Could you check a few things on this model? Use its own coordinates, in mm. A direction names the side the tool comes from. Coordinates: 2 decimals unless noted, no trailing zeros. Loops run counter-clockwise (first coordinate to the right, second up) from the corner with the lowest first, then second, coordinate; pieces in that order, holes last.
from build123d import *

# Parameters (mm, degrees)
SKETCH_1_R          = 3
SKETCH_1_R_2        = 1.5
EXTRUDE_1_DEPTH     = 25
EXTRUDE_2_DEPTH     = 5
SKETCH_3_R          = 1.5
CUT_EXTRUDE_1_DEPTH = 26
SKETCH_4_R          = 5
CUT_EXTRUDE_2_DEPTH = 4
SKETCH_5_R          = 1.5
EXTRUDE_3_DEPTH     = 5
SKETCH_6_R          = 5
CUT_EXTRUDE_3_DEPTH = 4
SKETCH_7_W          = 8
SKETCH_7_H          = 3
CUT_EXTRUDE_4_DEPTH = 25
SKETCH_8_R          = 1.5
CUT_EXTRUDE_5_DEPTH = 26
SKETCH_9_W          = 62.045271576
SKETCH_9_H          = 47.186533399
CUT_EXTRUDE_6_DEPTH = 2
SKETCH_10_R         = 43.321303534
CUT_EXTRUDE_7_DEPTH = 2


with BuildPart() as part:
    # 草图1 → 凸台-拉伸1 (new body)
    with BuildSketch(Plane.XY):
        with BuildLine():
            Line((-60, -3), (0, -3))
            ThreePointArc((0, -3), (-2.93041003, -0.642415018), (-1.255026274, 2.72486863))
            Line((-1.255026274, 2.72486863), (-5, 1))
            Line((-5, 1), (-60, 1))
            Line((-60, 1), (-60, -3))
        make_face()
        Circle(SKETCH_1_R)
        Circle(SKETCH_1_R_2, mode=Mode.SUBTRACT)
    extrude(amount=EXTRUDE_1_DEPTH)

    # 草图2 → 凸台-拉伸2 (add)
    with BuildSketch(Plane.XY.offset(25)):
        with BuildLine():
            Line((-60, -3), (-60, -19))
            Line((-60, -19), (-48, -19))
            Line((-48, -19), (-48, -14))
            ThreePointArc((-48, -14), (-46.535533906, -10.464466094), (-43, -9))
            Line((-43, -9), (-38, -9))
            ThreePointArc((-38, -9), (-34.464466094, -10.464466094), (-33, -14))
            Line((-33, -14), (-33, -23))
            Line((-33, -23), (-15, -23))
            Line((-15, -23), (-15, -13))
            Line((-15, -13), (-5, -3))
            Line((-5, -3), (-60, -3))
        make_face()
    extrude(amount=-EXTRUDE_2_DEPTH)

    # 草图3 → 切除-拉伸1 (cut, through all)
    with BuildSketch(Plane.XY.offset(25)):
        with Locations((-55, -14)):
            Circle(SKETCH_3_R)
        with Locations((-23, -14)):
            Circle(SKETCH_3_R)
    extrude(amount=-CUT_EXTRUDE_1_DEPTH, mode=Mode.SUBTRACT)

    # 草图4 → 切除-拉伸2 (cut)
    with BuildSketch(Plane.XY.offset(25)):
        Circle(SKETCH_4_R)
    extrude(amount=-CUT_EXTRUDE_2_DEPTH, mode=Mode.SUBTRACT)

    # 草图5 → 凸台-拉伸3 (add)
    with BuildSketch(Plane(origin=(0, 0, 0), x_dir=(-1, 0, 0), z_dir=(0, 0, -1))):
        with BuildLine():
            Line((60, -3), (5, -3))
            Line((5, -3), (15, -13))
            Line((15, -13), (15, -23))
            Line((15, -23), (33, -23))
            Line((33, -23), (33, -14))
            ThreePointArc((33, -14), (34.464466094, -10.464466094), (38, -9))
            Line((38, -9), (43, -9))
            ThreePointArc((43, -9), (46.535533906, -10.464466094), (48, -14))
            Line((48, -14), (48, -19))
            Line((48, -19), (60, -19))
            Line((60, -19), (60, -3))
        make_face()
        with Locations((23, -14)):
            Circle(SKETCH_5_R, mode=Mode.SUBTRACT)
        with Locations((55, -14)):
            Circle(SKETCH_5_R, mode=Mode.SUBTRACT)
    extrude(amount=-EXTRUDE_3_DEPTH)

    # 草图6 → 切除-拉伸3 (cut)
    with BuildSketch(Plane(origin=(0, 0, 0), x_dir=(-1, 0, 0), z_dir=(0, 0, -1))):
        Circle(SKETCH_6_R)
    extrude(amount=-CUT_EXTRUDE_3_DEPTH, mode=Mode.SUBTRACT)

    # 草图7 → 切除-拉伸4 (cut, through all)
    with BuildSketch(Plane(origin=(0, 1, 0), x_dir=(1, 0, 0), z_dir=(0, 1, 0))):
        with Locations((-56, -6.5)):
            Rectangle(SKETCH_7_W, SKETCH_7_H)
        with Locations((-56, -18.5)):
            Rectangle(SKETCH_7_W, SKETCH_7_H)
    extrude(amount=-CUT_EXTRUDE_4_DEPTH, mode=Mode.SUBTRACT)

    # 草图8 → 切除-拉伸5 (cut, through all)
    with BuildSketch(Plane(origin=(0, 0, 0), x_dir=(-1, 0, 0), z_dir=(0, 0, -1))):
        with Locations((58, -1)):
            Circle(SKETCH_8_R)
    extrude(amount=-CUT_EXTRUDE_5_DEPTH, mode=Mode.SUBTRACT)

    # 草图9 → 切除-拉伸6 (cut)
    with BuildSketch(Plane(origin=(0, 0, 0), x_dir=(-1, 0, 0), z_dir=(0, 0, -1))):
        with Locations((33.21865334, -9.347420282)):
            Rectangle(SKETCH_9_W, SKETCH_9_H)
    extrude(amount=-CUT_EXTRUDE_6_DEPTH, mode=Mode.SUBTRACT)

    # 草图10 → 切除-拉伸7 (cut)
    with BuildSketch(Plane.XY.offset(25)):
        with Locations((-29.013307515, -5.864856676)):
            Circle(SKETCH_10_R)
    extrude(amount=-CUT_EXTRUDE_7_DEPTH, mode=Mode.SUBTRACT)


solid = part.part
(1) Imagine slicing it at A-A, the plane x = -58. Write out the boundary of the cut face in (y, z).
Answers:
outline: (-19, 2) - (-2.5, 2) - (-2.5, 5) - (-19, 5) - close; (-19, 20) - (-2.5, 20) - (-2.5, 23) - (-19, 23) - close; (-3, 8) - (-2.5, 8) - (-2.5, 17) - (-3, 17) - close; (0.5, 2) - (1, 2) - (1, 5) - (0.5, 5) - close; (0.5, 8) - (1, 8) - (1, 17) - (0.5, 17) - close; (0.5, 20) - (1, 20) - (1, 23) - (0.5, 23) - close
(2) Which directions (+Z, -Z, +X, -X, +Y, -Y) give clear straight access to the entire face, cutting with the end or side of a thin tool? Please do faces 4 (the face through (-4.878, -1.1, 2.986)), 5 (the face through (-47, -11, 22)), 6 (the face through (-55, -1, 17)), 7 (the face through (-4.9, -1, 22)), 8 (the face through (-32, 1, 12)).
Answers:
face 4: -Z, +X
face 5: +Z, -Z, -Y
face 6: -X, +Y, -Y
face 7: +Z, +X
face 8: +Z, -Z, -X, +Y
(3) For pin 1 (2.5 mm diameter, centred on y = -17.5, z = 21, fed in from +X); pin 2 (3.5 mm diameter, centred on x = -52.5, z = 21, fed in from -Y); pin 3 (3 mm diameter, centred on x = -40.5, z = 19, fed in from +Y), each with a flat end and sliding along its axis, tell me the tip position at first contact or that it passes through.
Answers:
pin 1: stops at x = -15
pin 2: stops at y = -19
pin 3: stops at y = 1
(4) Imagine slicing it at C-C, the plane z = 14.25. Write out the boundary of the cut face in (x, y), and give its area (3 significant figures).
Answers:
outline: (-60, -3) - (0, -3) arc R3 ccw (long way) to (-1.26, 2.72) - (-5, 1) - (-60, 1) - close; hole circle Ø3 at (-58, -1); hole circle Ø3 at (0, 0)
area: 246 mm2
(5) Imagine slicing it at D-D, the plane x = -39.5. Write out the boundary of the cut face in (y, z).
Answers:
outline: (-9, 2) - (1, 2) - (1, 23) - (-9, 23) - (-9, 20) - (-3, 20) - (-3, 5) - (-9, 5) - close
(6) I need wall thicknesses on probe 1 along Z at (x, y) = (-25.5, -16.5); probe 2 along Y at (x, z) = (-55, 3.6); probe 3 along X at (y, z) = (-0.5, 9). Which ranges of each line are inside material? Lowest first, please.
Answers:
probe 1: z = 2 to 5, 20 to 23
probe 2: y = -19 to -15.5, -12.5 to 1
probe 3: x = -60 to -59.41, -56.59 to -1.41, 1.41 to 2.96
(7) We'd pull the mould along Y, two halves only. Please class faces 1 (the face through (-35, -10, 22)), 2 (the face through (-32, -8, 2)), 3 (the face through (-56.43, -13.55, 3.48)): +Y half, -Y half, draft (parallel to the pull), parting line (faces both ways), or undercut.
Answers:
face 1: -Y half
face 2: draft
face 3: undercut
(8) Imagine slicing it at B-B, the plane x = -23. Write out the boundary of the cut face in (y, z).
Answers:
outline: (-23, 2) - (-15.5, 2) - (-15.5, 5) - (-23, 5) - close; (-23, 20) - (-15.5, 20) - (-15.5, 23) - (-23, 23) - close; (-12.5, 2) - (1, 2) - (1, 23) - (-12.5, 23) - (-12.5, 20) - (-3, 20) - (-3, 5) - (-12.5, 5) - close
